Input: part model. Units: mm. Frame: model coordinates. A direction names the side the tool comes from. Round coordinates to 2 decimals unless told otherwise and drop trailing zeros. Write each loop counter-clockwise with the first axis right and the second up, starting at its lowest first coordinate (ties: lowest second). Pieces come first, ordered by that corner, then holes. Notation, with made-up numbers: (-6.75, 57) -> (-1.75, 57) arc R20 cw to (-1.75, 73) -> close; hole circle Ø9 at (12, 29.5). An arc over 180 degrees is marked (long way). Write item = value, one per line.
```python
from build123d import *

# Parameters (mm, degrees)
BOSS_EXTRUDE1_DEPTH = 4.7625


with BuildPart() as part:
    # Sketch1 → Boss-Extrude1 (new body)
    with BuildSketch(Plane.XY):
        with BuildLine():
            ThreePointArc((0.13375119, -12.340042072), (1.193950707, -11.485860744), (1.798906697, -10.266157088))
            Line((1.798906697, -10.266157088), (2.398140588, -7.862761221))
            ThreePointArc((2.398140588, -7.862761221), (2.461635419, -7.64822635), (2.543491476, -7.440004377))
            ThreePointArc((2.543491476, -7.440004377), (3.61061, -6.253759966), (5.171487057, -5.922730421))
            ThreePointArc((5.171487057, -5.922730421), (5.392740604, -5.955951983), (5.610280667, -6.008231282))
            Line((5.610280667, -6.008231282), (7.991299489, -6.690977442))
            ThreePointArc((7.991299489, -6.690977442), (9.350071835, -6.776922016), (10.619914323, -6.285852964))
            ThreePointArc((10.619914323, -6.285852964), (10.714040096, -6.185753934), (10.753665513, -6.054189108))
            ThreePointArc((10.753665513, -6.054189108), (10.544022542, -4.708938729), (9.790206185, -3.575179646))
            Line((9.790206185, -3.575179646), (8.008421255, -1.854529939))
            ThreePointArc((8.008421255, -1.854529939), (7.854376023, -1.692274367), (7.714978533, -1.517273956))
            ThreePointArc((7.714978533, -1.517273956), (7.22122, 0), (7.714978533, 1.517273956))
            ThreePointArc((7.714978533, 1.517273956), (7.854376023, 1.692274367), (8.008421255, 1.854529939))
            Line((8.008421255, 1.854529939), (9.790205754, 3.575179229))
            ThreePointArc((9.790205754, 3.575179229), (10.544022434, 4.708938449), (10.753665513, 6.054189108))
            ThreePointArc((10.753665513, 6.054189108), (10.714040096, 6.185753934), (10.619914323, 6.285852964))
            ThreePointArc((10.619914323, 6.285852964), (9.350071835, 6.776922015), (7.991299489, 6.690977442))
            Line((7.991299489, 6.690977442), (5.610280667, 6.008231282))
            ThreePointArc((5.610280667, 6.008231282), (5.392740604, 5.955951983), (5.171487057, 5.922730421))
            ThreePointArc((5.171487057, 5.922730421), (3.61061, 6.253759966), (2.543491476, 7.440004377))
            ThreePointArc((2.543491476, 7.440004377), (2.461635419, 7.64822635), (2.398140588, 7.862761221))
            Line((2.398140588, 7.862761221), (1.798906697, 10.266157088))
            ThreePointArc((1.798906697, 10.266157088), (1.193950707, 11.485860744), (0.13375119, 12.340042072))
            ThreePointArc((0.13375119, 12.340042072), (0, 12.371507867), (-0.13375119, 12.340042072))
            ThreePointArc((-0.13375119, 12.340042072), (-1.193950707, 11.485860744), (-1.798906697, 10.266157088))
            Line((-1.798906697, 10.266157088), (-2.398140588, 7.862761221))
            ThreePointArc((-2.398140588, 7.862761221), (-2.461635419, 7.64822635), (-2.543491476, 7.440004377))
            ThreePointArc((-2.543491476, 7.440004377), (-3.61061, 6.253759966), (-5.171487057, 5.922730421))
            ThreePointArc((-5.171487057, 5.922730421), (-5.392740604, 5.955951983), (-5.610280667, 6.008231282))
            Line((-5.610280667, 6.008231282), (-7.991299489, 6.690977442))
            ThreePointArc((-7.991299489, 6.690977442), (-9.350071835, 6.776922016), (-10.619914323, 6.285852964))
            ThreePointArc((-10.619914323, 6.285852964), (-10.714040096, 6.185753934), (-10.753665513, 6.054189108))
            ThreePointArc((-10.753665513, 6.054189108), (-10.544022542, 4.708938729), (-9.790206185, 3.575179646))
            Line((-9.790206185, 3.575179646), (-8.008421255, 1.854529939))
            ThreePointArc((-8.008421255, 1.854529939), (-7.854376023, 1.692274367), (-7.714978533, 1.517273956))
            ThreePointArc((-7.714978533, 1.517273956), (-7.22122, 0), (-7.714978533, -1.517273956))
            ThreePointArc((-7.714978533, -1.517273956), (-7.854376023, -1.692274367), (-8.008421255, -1.854529939))
            Line((-8.008421255, -1.854529939), (-9.790205754, -3.575179229))
            ThreePointArc((-9.790205754, -3.575179229), (-10.544022434, -4.708938449), (-10.753665513, -6.054189108))
            ThreePointArc((-10.753665513, -6.054189108), (-10.714040096, -6.185753934), (-10.619914323, -6.285852964))
            ThreePointArc((-10.619914323, -6.285852964), (-9.350071835, -6.776922015), (-7.991299489, -6.690977442))
            Line((-7.991299489, -6.690977442), (-5.610280667, -6.008231282))
            ThreePointArc((-5.610280667, -6.008231282), (-5.392740604, -5.955951983), (-5.171487057, -5.922730421))
            ThreePointArc((-5.171487057, -5.922730421), (-3.61061, -6.253759966), (-2.543491476, -7.440004377))
            ThreePointArc((-2.543491476, -7.440004377), (-2.461635419, -7.64822635), (-2.398140588, -7.862761221))
            Line((-2.398140588, -7.862761221), (-1.798906697, -10.266157088))
            ThreePointArc((-1.798906697, -10.266157088), (-1.193950707, -11.485860744), (-0.13375119, -12.340042072))
            ThreePointArc((-0.13375119, -12.340042072), (0, -12.371507867), (0.13375119, -12.340042072))
        make_face()
        with BuildLine():
            Line((1.313392554, -1.475), (-1.313392554, -1.475))
            ThreePointArc((-1.313392554, -1.475), (0, 1.975), (1.313392554, -1.475))
        make_face(mode=Mode.SUBTRACT)
    extrude(amount=BOSS_EXTRUDE1_DEPTH)


solid = part.part
```
1) First-contact query: P1, Ø1, axis at x = 4, z = 3, coming from the -Y side; P2, Ø2, axis at x = 8, z = 3, coming from the +Y side; P3, Ø1.5, axis at y = -9.5, z = 2.5, coming from the +X side; P4, Ø1, axis at x = 5, y = -8, coming from the +Z side. Flat tips, straight axial feed; report the tip coordinate or a pass-through.
Solutions:
P1 = -6.32
P2 = 6.81
P3 = 2.18
P4 = through
2) Draft query along X for faces 6 (the face through (1.18, -11.5, 2.35)), 7 (the face through (-1.206, -11.471, 2.348)), 8 (the face through (-6.784, 6.345, 2.348)). Return one class per face: +X half, -X half, draft (parallel to the pull), parting line (faces both ways), or undercut.
Solutions:
face_6 = +X half
face_7 = -X half
face_8 = undercut
3) Cut plane A-A (y = 0). Return the cut outline in (x, z) (1 decimal), and give its area (3 significant figures).
Solutions:
outline = (-7.2, 0) -> (-2, 0) -> (-2, 4.8) -> (-7.2, 4.8) -> close; (2, 0) -> (7.2, 0) -> (7.2, 4.8) -> (2, 4.8) -> close
area = 50.0 mm^2
4) Cut plane C-C (x = 3.5). Return the cut outline in (y, z), and give its area (3 significant figures).
Solutions:
outline = (-6.32, 0) -> (6.32, 0) -> (6.32, 4.76) -> (-6.32, 4.76) -> close
area = 60.2 mm^2
5) Access query for faces 1 (the face through (2.094, -9.081, 2.348)), 2 (the face through (6.817, 6.354, 2.348)), 3 (the face through (-10.55, 4.73, 2.35)), 4 (the face through (-6.817, -6.354, 2.348)), 5 (the face through (1.206, 11.471, 2.348)). Directions: +Z, -Z, +X, -X, +Y, -Y. A direction counts if a zero-diameter tool reaches every point of the face in a straight line with its end or side. Return the directions, or none.
Solutions:
face_1 = +Z, -Z, +X, -Y
face_2 = +Z, -Z, +Y
face_3 = +Z, -Z, -X
face_4 = +Z, -Z, -Y
face_5 = +Z, -Z, +X, +Y
6) Cut plane B-B (x = -0.75). Return the cut outline in (y, z) (1 decimal).
Solutions:
outline = (-11.9, 0) -> (-1.5, 0) -> (-1.5, 4.8) -> (-11.9, 4.8) -> close; (1.8, 0) -> (11.9, 0) -> (11.9, 4.8) -> (1.8, 4.8) -> close
7) Line query: L1, parallel to Y at x = 0, z = 1.5 (1 decimal); L2, parallel to Y at x = -1, z = 4.55 (3 decimals); L3, parallel to Y at x = -5, z = 0.35. Output: solid intervals per line, ascending. Write a range as from..to.
Solutions:
L1 = -12.4..-1.5, 2..12.4
L2 = -11.706..-1.475, 1.703..11.706
L3 = -5.91..5.91
